```python
from build123d import *

# Parameters (mm, degrees)
PAD_DEPTH       = 5
SKETCH001_W     = 65
SKETCH001_H     = 90
PAD001_DEPTH    = 9.75
SKETCH002_W     = 54.25
SKETCH002_H     = 90
POCKET_DEPTH    = 9.75
POCKET001_DEPTH = 9.75
SKETCH004_R     = 2.65
POCKET002_DEPTH = 5


with BuildPart() as part:
    # Sketch → Pad (new body)
    with BuildSketch(Plane.XY):
        Polygon((-32.5, 35), (-45, 35), (-45, 45), (45, 45), (45, 35), (32.5, 35), (32.5, -35), (45, -35), (45, -45), (-45, -45), (-45, -35), (-32.5, -35), align=None)
    extrude(amount=PAD_DEPTH)

    # Sketch001 (on Face14 of Pad) → Pad001 (join)
    with BuildSketch(Plane.XY.offset(5)):
        Rectangle(SKETCH001_W, SKETCH001_H)
    extrude(amount=PAD001_DEPTH)

    # Sketch002 (on Face19 of Pad001) → Pocket (cut)
    with BuildSketch(Plane.XY.offset(14.75)):
        Rectangle(SKETCH002_W, SKETCH002_H)
    extrude(amount=-POCKET_DEPTH, mode=Mode.SUBTRACT)

    # Sketch003 (on Face19 of Pocket) → Pocket001 (cut)
    with BuildSketch(Plane.XY.offset(14.75)):
        Polygon((-27.125, -2.05), (-28.575, -2.125), (-28.575, 2.125), (-27.125, 2.05), align=None)
    extrude(amount=-POCKET001_DEPTH, mode=Mode.SUBTRACT)

    # Sketch004 (on Face16 of Pocket001) → Pocket002 (cut)
    with BuildSketch(Plane.XY.offset(5)):
        with Locations((-40, 40)):
            Circle(SKETCH004_R)
        with Locations((40, 40)):
            Circle(SKETCH004_R)
        with Locations((40, -40)):
            Circle(SKETCH004_R)
        with Locations((-40, -40)):
            Circle(SKETCH004_R)
    extrude(amount=-POCKET002_DEPTH, mode=Mode.SUBTRACT)


solid = part.part
```
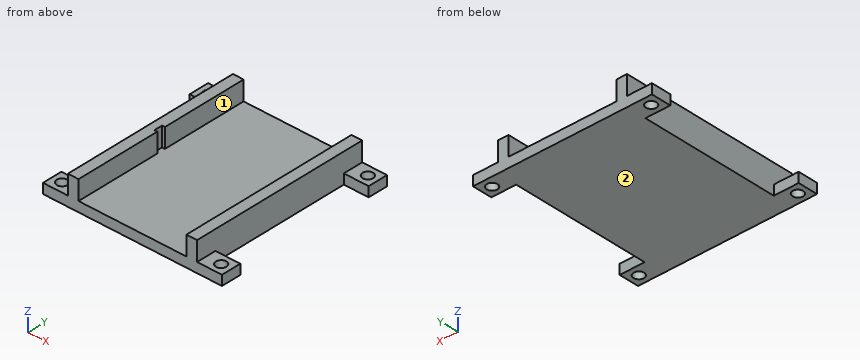
Could you check a few things on this model? Use its own coordinates, in mm. Face numbers are marked on the shaded views. Give positions to 0.01 mm unless a question says otherwise; leave off trailing zeros. Loops run counter-clockwise (first coordinate to the right, second up) from the corner with the lowest first, then second, coordinate; pieces in that order, holes last. Notation, with made-up numbers: (-24.5, -39.5) -> (26.5, -39.5) arc R11 ccw to (26.5, -28.5) -> close; hole circle Ø5 at (7, -21). An arc over 180 degrees is marked (long way). Put each result on its own line as item: value.
(1) Please list where these lines run through material, in increasing order: probe 1 along Y at (x, z) = (40, 3.35); probe 2 along X at (y, z) = (0.5, 7.75) (3 decimals); probe 3 along X at (y, z) = (15, 6.5) (3 decimals). Write a range as [from, to].
Computed:
probe 1: [-45, -42.65], [-37.35, -35], [35, 37.35], [42.65, 45]
probe 2: [-32.5, -28.575], [27.125, 32.5]
probe 3: [-32.5, -27.125], [27.125, 32.5]
(2) Imagine slicing it at C-C on y = -24.5. Write out the boundary of the cut face in (x, z) (3 decimals).
Computed:
outline: (-32.5, 0) -> (32.5, 0) -> (32.5, 14.75) -> (27.125, 14.75) -> (27.125, 5) -> (-27.125, 5) -> (-27.125, 14.75) -> (-32.5, 14.75) -> close
(3) Imagine slicing it at A-A on z = 9.25. Write out the boundary of the cut face in (x, y) (3 decimals), plus the area to 3 significant figures.
Computed:
outline: (-32.5, -45) -> (-27.125, -45) -> (-27.125, -2.05) -> (-28.575, -2.125) -> (-28.575, 2.125) -> (-27.125, 2.05) -> (-27.125, 45) -> (-32.5, 45) -> close; (27.125, -45) -> (32.5, -45) -> (32.5, 45) -> (27.125, 45) -> close
area: 961 mm^2
(4) Imagine slicing it at B-B on x = 40. Write out the boundary of the cut face in (y, z), plus the area to 3 significant figures.
Computed:
outline: (-45, 0) -> (-42.65, 0) -> (-42.65, 5) -> (-45, 5) -> close; (-37.35, 0) -> (-35, 0) -> (-35, 5) -> (-37.35, 5) -> close; (35, 0) -> (37.35, 0) -> (37.35, 5) -> (35, 5) -> close; (42.65, 0) -> (45, 0) -> (45, 5) -> (42.65, 5) -> close
area: 47.0 mm^2
(5) Imagine slicing it at D-D on z = 2.25. Write out the boundary of the cut face in (x, y), plus the area to 3 significant figures.
Computed:
outline: (-45, -45) -> (45, -45) -> (45, -35) -> (32.5, -35) -> (32.5, 35) -> (45, 35) -> (45, 45) -> (-45, 45) -> (-45, 35) -> (-32.5, 35) -> (-32.5, -35) -> (-45, -35) -> close; hole circle Ø5.3 at (-40, -40); hole circle Ø5.3 at (-40, 40); hole circle Ø5.3 at (40, -40); hole circle Ø5.3 at (40, 40)
area: 6,260 mm^2
(6) Thinking about a two-plate mould opening in X: for the marked faces 1 and 2, which applies, pulls with the +X half, pulls with the -X half, needs draft (parallel to the pull), parting line crosses it, or undercut?
Computed:
face 1: undercut
face 2: needs draft
(7) I'm going to push flat-ended pins straight in: pin 1 Ø8 at (y, z) = (-5.5, 8) entering from -X; pin 2 Ø1.3 at (y, z) = (0, 9.5) entering from +X; pin 3 Ø3 at (x, y) = (40, 40) entering from -Z; pin 4 Ø3 at (x, y) = (-37.5, -41.5) entering from +Z. Where does each tip first touch, or does it pass through?
Computed:
pin 1: x = -32.5
pin 2: x = 32.5
pin 3: through
pin 4: z = 5
